Design review of the part built by this model. Coordinates are the model's own, in mm. A direction names the side the tool comes from. Give positions to 0.01 mm unless a question says otherwise; leave off trailing zeros. Write each loop counter-clockwise with the first axis right and the second up, starting at its lowest first coordinate (ties: lowest second). Pieces come first, ordered by that corner, then holes. Notation, with made-up numbers: (-32, 30) -> (-4, 30) arc R17 cw to (-4, 63) -> close; hole circle Ø9 at (7, -39.5). An arc over 180 degrees is marked (long way). Use CSV: the item, a comma, the result in double quotes.
Autodesk Inventor part; units mm, degrees
ref_plane "YZ Plane" through (0, 0, 0) normal (1, 0, 0) x (0, 1, 0)
ref_plane "XZ Plane" through (0, 0, 0) normal (0, 1, 0) x (-1, 0, 0)
ref_plane "XY Plane" through (0, 0, 0) normal (0, 0, 1) x (1, 0, 0)
sketch "Sketch1" plane through (0, 0, 0) normal (0, 1, 0) x (-1, 0, 0)
  line L0 (-16.7648, -6.8244) -> (19.5108, -6.8244) construction
  line L1 (19.5108, -6.8244) -> (19.5108, -28.8158) construction
  line L2 (19.5108, -28.8158) -> (-16.7648, -28.8158) construction
  line L3 (-16.7648, -28.8158) -> (-16.7648, -6.8244) construction
  line L4 (6.77, 0) -> (-6.77, 0) construction
  line L5 (6.77, 2) -> (-6.77, 2)
  line L6 (-6.77, -2) -> (6.77, -2)
  arc A0 (6.77, -2) -> (6.77, 2) centre (6.77, 0) ccw
  arc A1 (-6.77, 2) -> (-6.77, -2) centre (-6.77, 0) ccw
  point P0 (0, 0)
  point P1 (-8.77, 0)
  point P2 (8.77, 0)
  dimension "d11" = 17.54
  dimension "d18" = 4
extrude "Extrusion1" add sketch "Sketch1" along normal blind 2
sketch "Sketch2" plane through (0, 2, 0) normal (0, 1, 0) x (1, 0, 0)
  arc A0 (6.77, -2) -> (6.77, 2) centre (6.77, 0) ccw
  line L0 (6.77, 2) -> (-6.77, 2)
  arc A1 (-6.77, 2) -> (-6.77, -2) centre (-6.77, 0) ccw
  line L1 (-6.77, -2) -> (6.77, -2)
  line L2 (-9.5, 0) -> (9.5, 0) construction
  line L3 (-9.5, -2) -> (9.5, -2)
  line L4 (9.5, 2) -> (-9.5, 2)
  arc A2 (-9.5, 2) -> (-9.5, -2) centre (-9.5, 0) ccw
  arc A3 (9.5, -2) -> (9.5, 2) centre (9.5, 0) ccw
  circle A4 centre (-10.22, 0) radius 0.75
  line L5 (0, -2) -> (0, 2)
  circle A5 centre (10.22, 0) radius 0.75
  point P0 (0, 0)
  point P1 (11.5, 0)
  point P2 (-11.5, 0)
  point P3 (0, 0)
  point P4 (-6.77, -2)
  point P5 (6.77, -2)
  dimension "d23" = 4
  dimension "d24" = 23
  dimension "d25" = 1.5
  dimension "d26" = 20.44
extrude "Extrusion2" add sketch "Sketch2" along normal blind 1
sketch "Sketch3" plane through (0, 3, 0) normal (0, 1, 0) x (1, 0, 0)
  line L0 (9.5, 2) -> (-9.5, 2)
  arc A0 (-9.5, 2) -> (-9.5, -2) centre (-9.5, 0) ccw
  line L1 (-9.5, -2) -> (9.5, -2)
  arc A1 (9.5, -2) -> (9.5, 2) centre (9.5, 0) ccw
  circle A2 centre (-10.22, 0) radius 0.75
  circle A3 centre (10.22, 0) radius 0.75
  line L2 (-9.5, 1.5) -> (9.5, 1.5)
  arc A4 (9.5, -1.5) -> (9.5, 1.5) centre (9.5, 0) ccw
  line L3 (9.5, -1.5) -> (-9.5, -1.5)
  arc A5 (-9.5, 1.5) -> (-9.5, -1.5) centre (-9.5, 0) ccw
  point P0 (0, 0)
  dimension "d29" = 0.5
extrude "Extrusion3" add sketch "Sketch3" along normal blind 1 contours A1 L1 A0 L0
sketch "Sketch4" plane through (0, 0, 0) normal (0, -1, 0) x (1, 0, 0)
  circle A0 centre (-3.81, 0) radius 0.755
  circle A1 centre (-1.27, 0) radius 0.755
  line L0 (-6.77, 2) -> (6.77, 2)
  line L1 (0, 2) -> (0, -2)
  line L2 (6.77, -2) -> (-6.77, -2)
  circle A2 centre (3.81, 0) radius 0.755
  circle A3 centre (1.27, 0) radius 0.755
  point P0 (0, 0)
  dimension "d32" = 2.54
  dimension "d33" = 7.62
  dimension "d34" = 1.51
extrude "Extrusion4" cut sketch "Sketch4" against normal blind 1
sketch "Sketch5" plane through (-3.81, 1, 0) normal (0, -1, 0) x (1, 0, 0)
  circle A0 centre (0, 0) radius 0.755
  circle A1 centre (2.54, 0) radius 0.755
  circle A2 centre (5.08, 0) radius 0.755
  circle A3 centre (7.62, 0) radius 0.755
  circle A4 centre (0, 0) radius 0.755
  circle A5 centre (0, 0) radius 0.45
  circle A6 centre (2.54, 0) radius 0.45
  circle A7 centre (5.08, 0) radius 0.45
  circle A8 centre (7.62, 0) radius 0.45
  point P0 (3.81, 0)
  dimension "d37" = 0.9
extrude "Extrusion5" add sketch "Sketch5" along normal blind 2 contours A5 | A6 | A7 | A8
fillet "Fillet1" radius 0.45 4 edges at (-4.26, -1, 0) (-1.72, -1, 0) (0.82, -1, 0) (3.36, -1, 0)
sketch "Sketch6" plane through (0, 0, 0) normal (0, -1, 0) x (1, 0, 0)
  circle A0 centre (1.27, 0) radius 0.755
  circle A1 centre (-1.27, 0) radius 0.755
  circle A2 centre (3.81, 0) radius 0.755
  circle A3 centre (-3.81, 0) radius 0.755
  arc A4 (6.77, -2) -> (6.77, 2) centre (6.77, 0) ccw
  line L0 (-6.77, 2) -> (6.77, 2)
  arc A5 (-6.77, 2) -> (-6.77, -2) centre (-6.77, 0) ccw
  line L1 (6.77, -2) -> (-6.77, -2)
  circle A6 centre (-6.77, 0) radius 1.5
  circle A7 centre (6.77, 0) radius 1.5
  point P0 (0, 0)
  dimension "d41" = 3
extrude "Extrusion6" cut sketch "Sketch6" against normal blind 0.1 contours A6 | A7
properties part number "Connector1"
(1) Clearance check with flat-ended pins moving along their axes: pin 1 (2 mm diameter, centred on x = -10.22, z = 0, fed in from -Y); pin 2 (0.9 mm diameter, centred on x = 10.22, z = 0, fed in from +Y); pin 3 (2 mm diameter, centred on x = 9.5, z = 1, fed in from -Y); pin 4 (0.5 mm diameter, centred on x = 3.5, z = 0, fed in from -Y). State where each tip first meets the part, or that it passes through.
Established:
pin 1,"stops at y = 2"
pin 2,"passes through"
pin 3,"stops at y = 0"
pin 4,"stops at y = -1"
(2) Take a section at C-C (x = 10). Write out the cut boundary in (y, z), then the cut area to 3 significant figures.
Established:
outline,"(2, -1.94) -> (4, -1.94) -> (4, -1.41) -> (3, -1.41) -> (3, -0.72) -> (2, -0.72) -> close; (2, 0.72) -> (3, 0.72) -> (3, 1.41) -> (4, 1.41) -> (4, 1.94) -> (2, 1.94) -> close"
area,"3.48 mm2"
(3) Tool access review of faces 1 (the face through (-10.97, 2.49, 0.03)), 2 (the face through (-11, 3.5, 0)), 3 (the face through (8.77, 0.99, -0.04)), 4 (the face through (-8.77, 0.99, 0.04)), 5 (the face through (4.239, 0.236, -0.135)): name each direction out of +Z, -Z, +X, -X, +Y, -Y from which nothing blocks a thin tool from reaching the whole face with its end or side.
Established:
face 1,"+Y, -Y"
face 2,"+Y"
face 3,"+X, -Y"
face 4,"-X, -Y"
face 5,"-Y"
(4) Mouldability with a two-part tool opening along Z and no side actions: class faces 6 (the face through (0, 3, 0)), 7 (the face through (-11.5, 3, 0)), 8 (the face through (0, 2, 2)) as +Z half, -Z half, draft (parallel to the pull), parting line (faces both ways), or undercut.
Established:
face 6,"undercut"
face 7,"parting line"
face 8,"+Z half"
(5) Take a section at A-A (y = 0.75). State how many separate pieces and enclosed holes the cut face has, then the cut area to 3 significant figures.
Established:
separate pieces,"5"
enclosed holes,"4"
area,"62.1 mm2"
(6) Take a section at B-B (y = 3.45). Write out the cut boundary in (x, z).
Established:
outline,"(-9.5, -2) -> (9.5, -2) arc R2 ccw to (9.5, 2) -> (-9.5, 2) arc R2 ccw to start; hole (-9.5, -1.5) -> (9.5, -1.5) arc R1.5 ccw to (9.5, 1.5) -> (-9.5, 1.5) arc R1.5 ccw to start"
(7) For line 1 along X through (y, z) = (-0.35, 0.05); line 2 along Z through (x, y) = (1.27, 0.3) (3 decimals); line 3 along Y through (x, z) = (-8.5, 0.6), list the stretches that pass through material, from the lowest coordinate up. Write a range as [from, to].
Established:
line 1,"x = [-4.26, -3.36], [-1.72, -0.82], [0.82, 1.72], [3.36, 4.26]"
line 2,"z = [-2, -0.755], [-0.45, 0.45], [0.755, 2]"
line 3,"y = [0, 3]"
